Check sheet for the modelled part. Datum: model origin and axes. Units: mm. Round coordinates to 2 decimals unless told otherwise and drop trailing zeros. Loops run counter-clockwise (first coordinate to the right, second up) from the corner with the lowest first, then second, coordinate; pieces in that order, holes last. Notation, with made-up numbers: (-14, -12.75) -> (8, -12.75) arc R19 ccw to (8, 24.25) -> close; hole circle Ø4 at (-22, -11). An arc over 180 degrees is marked (long way). One line per question, with ' | ' between items.
Autodesk Inventor part; units mm, degrees
ref_plane "Work Plane2" through (-85, 0, 0) normal (1, 0, 0) x (0, 0, -1)
ref_plane "YZ Plane" through (0, 0, 0) normal (1, 0, 0) x (0, 1, 0)
ref_plane "XZ Plane" through (0, 0, 0) normal (0, 1, 0) x (-1, 0, 0)
sketch "Sketch1" plane through (0, 0, 0) normal (0, 1, 0) x (-1, 0, 0)
  line L0 (0, 0) -> (170, 0)
  line L1 (170, 0) -> (170, -160)
  line L2 (170, -160) -> (0, -160)
  line L3 (0, -160) -> (0, 0)
  line L4 (5, -5) -> (165, -5)
  line L5 (165, -5) -> (165, -155)
  line L6 (165, -155) -> (5, -155)
  line L7 (5, -155) -> (5, -5)
  line L8 (95, -5) -> (75, -5)
  line L9 (75, -5) -> (75, -155)
  line L10 (75, -155) -> (95, -155)
  line L11 (95, -155) -> (95, -5)
  point P0 (85, -5)
  point P1 (85, 0)
  point P2 (95, -155)
  point P3 (75, -5)
  dimension "d0" = 170
  dimension "d1" = 160
  dimension "d2" = 5
  dimension "d5" = 20
extrude "Extrusion1" add sketch "Sketch1" along normal blind 10 contours L0 L1 L2 L3 | L4 L11 L6 L9
fillet "Fillet1" radius 3 8 edges at (-165, 5, -5) (-95, 5, -5) (-5, 5, -5) (-5, 5, -155) (-75, 5, -155) (-95, 5, -155) (-75, 5, -5) (-165, 5, -155)
sketch "Sketch2" plane through (-5, 0, -152) normal (-1, 0, 0) x (0, 0, 1)
  line L0 (144, 10) -> (144, 0) construction
  line L1 (144, 5) -> (0, 5) construction
  line L2 (0, 0) -> (0, 10) construction
  line L3 (147, 0) -> (147, 10) construction
  line L4 (-3, 10) -> (-3, 0) construction
  point P0 (152, 0)
  point P1 (102, 5)
  point P2 (42, 5)
  point P3 (-3, 5)
  dimension "d20" = 45
  dimension "d21" = 45
hole "Hole1" at (-5, 5, -50) at (-5, 5, -110) direction (1, 0, 0) diameter 3.5 end through all
sketch "Sketch5" plane through (0, 0, 0) normal (1, 0, 0) x (0, 0, -1)
  line L0 (8, 10) -> (152, 10)
  line L1 (8, 0) -> (152, 0)
  line L2 (35, 10) -> (125, 10)
  line L3 (125, 10) -> (125, 0)
  line L4 (125, 0) -> (35, 0)
  line L5 (35, 0) -> (35, 10)
  line L6 (0, 0) -> (0, 10)
  point P0 (0, 5)
  dimension "d37" = 90
  dimension "d38" = 35
extrude "Extrusion5" cut sketch "Sketch5" against normal blind 2
sketch "Sketch6" plane through (-170, 0, -160) normal (-1, 0, 0) x (0, 0, 1)
  line L0 (8, 0) -> (152, 0)
  line L1 (125, 10) -> (35, 10)
  line L2 (35, 0) -> (125, 0)
  line L3 (125, 0) -> (125, 10)
  line L4 (125, 10) -> (35, 10)
  line L5 (35, 10) -> (35, 0)
  line L6 (0, 0) -> (0, 10)
  point P0 (160, 0)
  dimension "d41" = 90
  dimension "d42" = 35
extrude "Extrusion6" cut sketch "Sketch6" against normal blind 2
ref_plane "Work Plane2" through (-85, 0, 0) normal (1, 0, 0) x (0, 0, -1)
mirror "Mirror2" about plane through (-85, 0, 0) normal (1, 0, 0) of "Hole1"
properties part number "Mirror_shell3" material "Aluminum 6061"
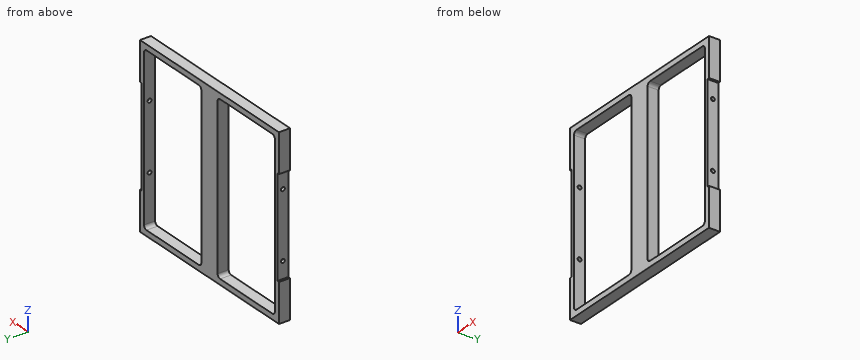
(1) Go/stop test with flat-tipped pins: pin 1 (3 mm diameter, centred on y = 5, z = -110, fed in from -X); pin 2 (5 mm diameter, centred on y = 7, z = -46, fed in from -X); pin 3 (2 mm diameter, centred on x = -168.5, y = 5, fed in from +Z); pin 4 (5.5 mm diameter, centred on y = 5, z = -50, fed in from +X). Record where each tip stops, or that it passes through.
Answer:
pin 1: stops at x = -95 | pin 2: stops at x = -168 | pin 3: stops at z = 0 | pin 4: stops at x = -2
(2) Scan lines: probe 1 along Z at (x, y) = (-2.9, 5); probe 2 along X at (y, z) = (3.25, -58); probe 3 along Y at (x, z) = (-167.4, -50). Record each from-to range of solid material in increasing order.
Answer:
probe 1: z = -160 to -111.75, -108.25 to -51.75, -48.25 to 0 | probe 2: x = -168 to -165, -95 to -75, -5 to -2 | probe 3: y = 0 to 3.25, 6.75 to 10
(3) Sectioned sample at D-D, the plane z = -83. Record the cut outline in (x, y).
Answer:
outline: (-168, 0) -> (-165, 0) -> (-165, 10) -> (-168, 10) -> close; (-95, 0) -> (-75, 0) -> (-75, 10) -> (-95, 10) -> close; (-5, 0) -> (-2, 0) -> (-2, 10) -> (-5, 10) -> close
(4) Sectioned sample at A-A, the plane z = -27. Record the cut outline in (x, y), and give its area (3 significant figures).
Answer:
outline: (-170, 0) -> (-165, 0) -> (-165, 10) -> (-170, 10) -> close; (-95, 0) -> (-75, 0) -> (-75, 10) -> (-95, 10) -> close; (-5, 0) -> (0, 0) -> (0, 10) -> (-5, 10) -> close | area: 300 mm2
(5) Sectioned sample at B-B, the plane x = -122. Record the cut outline in (y, z).
Answer:
outline: (0, -160) -> (10, -160) -> (10, -155) -> (0, -155) -> close; (0, -5) -> (10, -5) -> (10, 0) -> (0, 0) -> close
(6) Sectioned sample at C-C, the plane y = 5. Count the separate pieces of the cut face and the enclosed holes in it, and give its area (3 significant figures).
Answer:
separate pieces: 3 | enclosed holes: 0 | area: 5,810 mm2
